CAD build for the part. Positions are in the model's coordinates, mm. A direction names the side the tool comes from. Give positions to 0.01 mm unless a question says otherwise; leave off trailing zeros. Loops run counter-clockwise (first coordinate to the right, second up) from the corner with the lowest first, then second, coordinate; pieces in that order, holes last. Notation, with made-up numbers: (55.5, 62) -> (87.5, 62) arc R24 ccw to (87.5, 90) -> close; hole circle Ø7 at (-39.75, 38). An arc over 180 degrees is marked (long way). Use one line per item in the form item = value.
Autodesk Inventor part; units mm, degrees
ref_plane "Arbeitsebene1" through (0, 0, 4) normal (0, 0, 1) x (1, 0, 0)
ref_plane "Arbeitsebene2" through (0, 0, 26) normal (0, 0, 1) x (1, 0, 0)
ref_plane "YZ Plane" through (0, 0, 0) normal (1, 0, 0) x (0, 1, 0)
sketch "Skizze1" plane through (0, 0, 0) normal (0, 0, 1) x (1, 0, 0)
  line L0 (0, 0) -> (14, 0)
  line L1 (14, 0) -> (14, 8)
  line L2 (14, 8) -> (0, 8)
  line L3 (0, 8) -> (0, 0)
extrude "Extrusion1" add sketch "Skizze1" along normal blind 26
ref_plane "Arbeitsebene1" through (0, 0, 4) normal (0, 0, 1) x (1, 0, 0)
sketch "Skizze2" plane through (0, 0, 4) normal (0, 0, 1) x (1, 0, 0)
  line L0 (0, 0) -> (11.5, 0)
  line L1 (11.5, 0) -> (11.5, 6.25)
  line L2 (11.5, 6.25) -> (0, 6.25)
  line L3 (0, 6.25) -> (0, 0)
extrude "Extrusion2" cut sketch "Skizze2" against normal blind 22
ref_plane "Arbeitsebene2" through (0, 0, 26) normal (0, 0, 1) x (1, 0, 0)
sketch "Skizze3" plane through (0, 0, 26) normal (0, 0, 1) x (1, 0, 0)
  circle A0 centre (0, 0) radius 2.5
extrude "Extrusion3" cut sketch "Skizze3" against normal blind 4
sketch "Skizze4" plane through (0, 0, 0) normal (0, 0, 1) x (1, 0, 0)
  circle A0 centre (0, 0) radius 1
  circle A1 centre (14, 0) radius 1
extrude "Extrusion4" cut sketch "Skizze4" along normal blind 4
properties part number "Servo_Halterung"
1. Cut at A-A, the plane z = 3.25. Write the cut outline in (x, y), then the cut area to 3 significant figures.
Result sheet:
outline = (0, 6.25) -> (11.5, 6.25) -> (11.5, 0) -> (13, 0) arc R1 cw to (14, 1) -> (14, 8) -> (0, 8) -> close
area = 39.3 mm^2
2. Drop flat-ended pins along their axis: P1, Ø0.5, axis at x = 13.5, y = 0.5, coming from the -Z side; P2, Ø3, axis at y = 2.5, z = 1, coming from the -X side. Give the stop position or say it passes through.
Result sheet:
P1 = 4
P2 = 11.5
3. Drill centre lines: line 1 (X direction, y = 2.25, z = 2.25); line 2 (Z direction, x = 1.5, y = 3.75); line 3 (Y direction, x = 8.5, z = 2). Where is each one in solid material? Low to high.
Result sheet:
line_1 = 11.5 to 14
line_2 = 4 to 26
line_3 = 6.25 to 8
4. Cut at B-B, the plane x = 6. Write the cut outline in (y, z).
Result sheet:
outline = (0, 4) -> (6.25, 4) -> (6.25, 0) -> (8, 0) -> (8, 26) -> (0, 26) -> close
5. Cut at C-C, the plane y = 5.5. Write the cut outline in (x, z), then the cut area to 3 significant figures.
Result sheet:
outline = (0, 4) -> (11.5, 4) -> (11.5, 0) -> (14, 0) -> (14, 26) -> (0, 26) -> close
area = 318 mm^2
6. Tool access for faces 1 (the flat face through (11.5, 3, 2)), 2 (the flat face through (13.6, 0.4, 4)), 3 (the cylindrical face through (1.787, 1.748, 24.028)), 4 (the flat face through (10, 7, 0)), 5 (the flat face through (7, 0, 13)): list every direction of +Z, -Z, +X, -X, +Y, -Y with a clear straight run to the whole face (end or side of a thin tool).
Result sheet:
face_1 = -Z, -X, -Y
face_2 = -Z, +X, -Y
face_3 = +Z, -X, -Y
face_4 = -Z, +X, -X, +Y, -Y
face_5 = +Z, -Z, +X, -X, -Y
7. Cut at D-D, the plane y = 2.25. Write the cut outline in (x, z), then the cut area to 3 significant figures.
Result sheet:
outline = (0, 4) -> (11.5, 4) -> (11.5, 0) -> (14, 0) -> (14, 26) -> (1.09, 26) -> (1.09, 22) -> (0, 22) -> close
area = 314 mm^2
